The model under review builds one solid part; all positions refer to its coordinate system, in mm. A direction names the side the tool comes from. Round coordinates to 2 decimals unless told otherwise and drop trailing zeros. Order: outer loops, then holes, each group sorted by start corner. A loop starts at its lowest first (then second) coordinate and runs counter-clockwise, first axis right, second up.
1) Consider section B-B (z = 2.25). Give the boundary of the cut face in (x, y).
2) Consider section D-D (z = 6.75). Give the boundary of the cut face in (x, y), then the cut area to 3 significant figures.
3) Mouldability with a two-part tool opening along Y and no side actions: class faces 1 (the face through (0, 3, 0)), 2 (the face through (-4.68, 13.9, 4.22)), 3 (the face through (0, 0.45, 1.2)) as pulls with the +Y half, pulls with the -Y half, needs draft (parallel to the pull), parting line crosses it, or undercut.
4) Consider section A-A (x = 1.5). Give the boundary of the cut face in (y, z).
5) Machinability: for faces 4 (the face through (5, 0, 7)), 5 (the face through (-4.75, 0, 4)), 6 (the face through (0, 1, 1.5)), 7 (the face through (0, 5, 0.9)), 8 (the face through (-5.25, 5, 4)), which of the approach directions +Z, -Z, +X, -X, +Y, -Y give a long, thin tool a straight path to every point of the face, cutting with its end or side? Answer none if there is none.
6) Clearance check with flat-ended pins moving along their axes: P1, Ø0.5, axis at x = 1, z = 8, coming from the -Y side; P2, Ø4, axis at x = 1, y = 9.5, coming from the -Z side; P3, Ø0.5, axis at x = 1, y = 1, coming from the +Z side; P4, Ø5, axis at x = 0, z = 3.5, coming from the -Y side. State where each tip first meets the part, or that it passes through.
7) Consider section C-C (x = 0.25). Give the boundary of the cut face in (y, z), then the cut area to 3 significant figures.
8) To check wall thickness, follow L1, parallel to X at y = 7.25, z = 5.25; L2, parallel to Z at x = -1.25, y = 4.25; L3, parallel to Z at x = 1, y = 6.25. State the ranges of each line that lie inside material, in increasing order.
from build123d import *

# Parameters (mm, degrees)
F0_W     = 8.5
F0_H     = 11.400557369
F0_W_2   = 0.9711329822
F0_H_2   = 1.599442631
F0_W_3   = 1.0288670178
F1_DEPTH = 0.9
F2_DEPTH = 1.5
F3_DEPTH = 7
F5_W     = 10.5
F5_H     = 13
F6_DEPTH = 1.5
F7_R     = 2
F9_DEPTH = 0.9


# Not quite as in the source:
# - a feature names something its author has since deleted; it is built from what else it names


with BuildPart() as f1:
    # F0 (on Top) → F1 (new body)
    with BuildSketch(Plane.XY):
        with Locations((-0.0288670178, 7.2002786845)):
            Rectangle(F0_W, F0_H)
        Polygon((-5.25, 1.5), (-5.25, -1.5), (-4.2211329822, -1.5), (-4.2413398946, -0.45), (-4.75, -0.45), (-4.75, 0.45), (-4.2586601054, 0.45), (-4.2788670178, 1.5), align=None)
        Polygon((4.2211329822, 1.5), (-4.2788670178, 1.5), (-4.2586601054, 0.45), (4.2413398946, 0.45), align=None)
        with Locations((-4.7644335089, 7.2002786845)):
            Rectangle(F0_W_2, F0_H)
        Polygon((4.2586601054, -0.45), (4.2788670178, -1.5), (5.25, -1.5), (5.25, 1.5), (4.2211329822, 1.5), (4.2413398946, 0.45), (4.75, 0.45), (4.75, -0.45), align=None)
        Polygon((-4.2413398946, -0.45), (-4.2211329822, -1.5), (4.2788670178, -1.5), (4.2586601054, -0.45), align=None)
        Polygon((-4.2586601054, 0.45), (-4.2413398946, -0.45), (4.2586601054, -0.45), (4.2413398946, 0.45), align=None)
        Polygon((-4.75, -0.45), (-4.2413398946, -0.45), (-4.2586601054, 0.45), (-4.75, 0.45), align=None)
        Polygon((4.2413398946, 0.45), (4.2586601054, -0.45), (4.75, -0.45), (4.75, 0.45), align=None)
        with Locations((-4.7644335089, 13.7002786845)):
            Rectangle(F0_W_2, F0_H_2)
        with Locations((-0.0288670178, 13.7002786845)):
            Rectangle(F0_W, F0_H_2)
        with Locations((4.7355664911, 13.7002786845)):
            Rectangle(F0_W_3, F0_H_2)
        with Locations((4.7355664911, 7.2002786845)):
            Rectangle(F0_W_3, F0_H)
    extrude(amount=F1_DEPTH)

    # F0 (on Top) → F2 (join)
    with BuildSketch(Plane.XY):
        Polygon((-4.2413398946, -0.45), (-4.2211329822, -1.5), (4.2788670178, -1.5), (4.2586601054, -0.45), align=None)
        Polygon((-5.25, 1.5), (-5.25, -1.5), (-4.2211329822, -1.5), (-4.2413398946, -0.45), (-4.75, -0.45), (-4.75, 0.45), (-4.2586601054, 0.45), (-4.2788670178, 1.5), align=None)
        Polygon((4.2586601054, -0.45), (4.2788670178, -1.5), (5.25, -1.5), (5.25, 1.5), (4.2211329822, 1.5), (4.2413398946, 0.45), (4.75, 0.45), (4.75, -0.45), align=None)
        Polygon((4.2211329822, 1.5), (-4.2788670178, 1.5), (-4.2586601054, 0.45), (4.2413398946, 0.45), align=None)
        with Locations((-4.7644335089, 7.2002786845)):
            Rectangle(F0_W_2, F0_H)
        with Locations((-4.7644335089, 13.7002786845)):
            Rectangle(F0_W_2, F0_H_2)
        with Locations((-0.0288670178, 13.7002786845)):
            Rectangle(F0_W, F0_H_2)
        with Locations((4.7355664911, 13.7002786845)):
            Rectangle(F0_W_3, F0_H_2)
        with Locations((4.7355664911, 7.2002786845)):
            Rectangle(F0_W_3, F0_H)
    extrude(amount=F2_DEPTH)

    # F0 (on Top) → F3 (join)
    with BuildSketch(Plane.XY):
        Polygon((-5.25, 1.5), (-5.25, -1.5), (-4.2211329822, -1.5), (-4.2413398946, -0.45), (-4.75, -0.45), (-4.75, 0.45), (-4.2586601054, 0.45), (-4.2788670178, 1.5), align=None)
        Polygon((4.2586601054, -0.45), (4.2788670178, -1.5), (5.25, -1.5), (5.25, 1.5), (4.2211329822, 1.5), (4.2413398946, 0.45), (4.75, 0.45), (4.75, -0.45), align=None)
        with Locations((-4.7644335089, 13.7002786845)):
            Rectangle(F0_W_2, F0_H_2)
        with Locations((-0.0288670178, 13.7002786845)):
            Rectangle(F0_W, F0_H_2)
        with Locations((4.7355664911, 13.7002786845)):
            Rectangle(F0_W_3, F0_H_2)
        with Locations((-4.7644335089, 7.2002786845)):
            Rectangle(F0_W_2, F0_H)
        with Locations((4.7355664911, 7.2002786845)):
            Rectangle(F0_W_3, F0_H)
    extrude(amount=F3_DEPTH)

    # F5 (on offset) → F6 (join)
    with BuildSketch(Plane.XY.offset(7)):
        with Locations((0, 8)):
            Rectangle(F5_W, F5_H)
    extrude(amount=F6_DEPTH)

    # F7
    f7_edges = [f1.edges().sort_by_distance(p)[0] for p in [
        (5.25, 14.5, 4.25),
        (0, 14.5, 8.5),
        (5.25, 8, 8.5),
        (5.25, 6.5, 0),
        (0, 14.5, 0),
        (-5.25, 6.5, 0),
        (-5.25, 14.5, 4.25),
        (-5.25, 8, 8.5),
    ]]
    fillet(f7_edges, radius=F7_R)

    # F8 (on Top) → F9 (cut, through all)
    with BuildSketch(Plane.XY):
        with BuildLine():
            ThreePointArc((0, 5.75), (2.2980970389, 6.7019029611), (3.25, 9))
            ThreePointArc((3.25, 9), (-2.2980970389, 11.2980970389), (0, 5.75))
        make_face()
    extrude(amount=F9_DEPTH, mode=Mode.SUBTRACT)


solid = f1.part
Answer below:
1. outline: (-5.25, -1.5) - (-4.22, -1.5) - (-4.24, -0.45) - (-4.75, -0.45) - (-4.75, 0.45) - (-4.26, 0.45) - (-4.28, 1.5) - (-4.28, 12.9) - (4.22, 12.9) - (4.22, 1.5) - (4.24, 0.45) - (4.75, 0.45) - (4.75, -0.45) - (4.26, -0.45) - (4.28, -1.5) - (5.25, -1.5) - (5.25, 12.5) arc R2 ccw to (3.25, 14.5) - (-3.25, 14.5) arc R2 ccw to (-5.25, 12.5) - close
2. outline: (-5.23, -1.5) - (-4.22, -1.5) - (-4.24, -0.45) - (-4.75, -0.45) - (-4.75, 0.45) - (-4.26, 0.45) - (-4.28, 1.5) - (-4.28, 12.9) - (4.22, 12.9) - (4.22, 1.5) - (4.24, 0.45) - (4.75, 0.45) - (4.75, -0.45) - (4.26, -0.45) - (4.28, -1.5) - (5.23, -1.5) - (5.23, 12.5) arc R1.98 ccw to (3.25, 14.48) - (-3.25, 14.48) arc R1.98 ccw to (-5.23, 12.5) - close
2. area: 42.3 mm2
3. face 1: needs draft
3. face 2: pulls with the +Y half
3. face 3: undercut
4. outline: (-1.5, 0) - (6.12, 0) - (6.12, 0.9) - (1.5, 0.9) - (1.5, 1.5) - (0.45, 1.5) - (0.45, 0.9) - (-0.45, 0.9) - (-0.45, 1.5) - (-1.5, 1.5) - close; (1.5, 7) - (12.9, 7) - (12.9, 0.9) - (11.88, 0.9) - (11.88, 0) - (12.5, 0) arc R2 ccw to (14.5, 2) - (14.5, 6.5) arc R2 ccw to (12.5, 8.5) - (1.5, 8.5) - close
5. face 4: +Z, +X, -X, -Y
5. face 5: +Z
5. face 6: +Z, -Y
5. face 7: none
5. face 8: +Z, -Z, -X, +Y, -Y
6. P1: stops at y = 1.5
6. P2: stops at z = 7
6. P3: stops at z = 1.5
6. P4: stops at y = -1.5
7. outline: (-1.5, 0) - (5.76, 0) - (5.76, 0.9) - (1.5, 0.9) - (1.5, 1.5) - (0.45, 1.5) - (0.45, 0.9) - (-0.45, 0.9) - (-0.45, 1.5) - (-1.5, 1.5) - close; (1.5, 7) - (12.9, 7) - (12.9, 0.9) - (12.24, 0.9) - (12.24, 0) - (12.5, 0) arc R2 ccw to (14.5, 2) - (14.5, 6.5) arc R2 ccw to (12.5, 8.5) - (1.5, 8.5) - close
7. area: 37.4 mm2
8. L1: x = -5.25 to -4.28, 4.22 to 5.25
8. L2: z = 0 to 0.9, 7 to 8.5
8. L3: z = 7 to 8.5
